For this review, take the finished solid that the model builds, in its own axes (mm). Face numbers are marked on the shaded views. Round coordinates to 2 decimals unless told otherwise and drop trailing zeros. Order: outer loops, then holes, each group sorted by start corner. A loop starts at its lowest first (then second) coordinate and runs counter-clockwise, first axis right, second up. Notation, with made-up numbers: (18, -9) -> (43, -9) arc R16 cw to (43, 14) -> close; hole circle Ø5 at (50, 34.5). An arc over 180 degrees is marked (long way). Use a Markdown table: item, result. Add a question column.
1) Consider section C-C (x = 6.8). State the section outline as (y, z) points, plus the area to 3 significant figures.
2) Consider section D-D (z = 13). State the section outline as (x, y) points.
3) Draft analysis for pull direction X (two halves, no side actions). For the marked faces 1, 2 and 3, state which applies: pulls with the +X half, pulls with the -X half, needs draft (parallel to the pull), parting line crosses it, or undercut.
4) Consider section B-B (y = 1.35). State the section outline as (x, z) points.
5) Wall thickness on line 1 along Z through (x, y) = (8, 1.65); line 2 along Z through (x, y) = (5, 2.5); line 3 along Z through (x, y) = (5.5, 0.5): over which ranges is each line inside the solid? List them lowest first. Write a range as [from, to].
6) Clearance check with a flat-ended pin moving along its axis: P1, Ø1.8, axis at x = 7.3, z = 7.68, coming from the +Y side. State where the tip first meets the part, or that it passes through.
7) Consider section A-A (z = 18.32). State the section outline as (x, y) points.
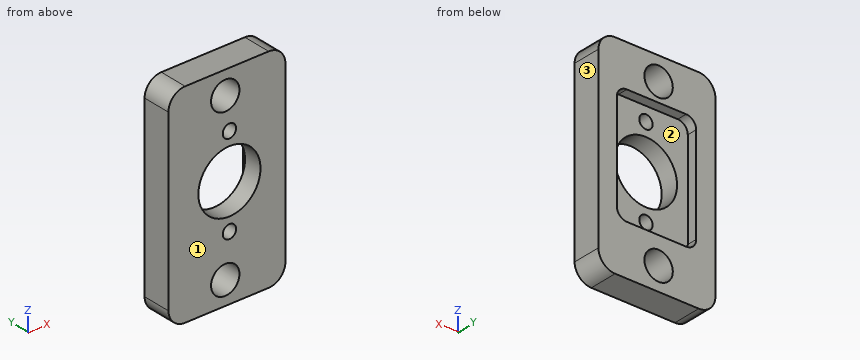
```python
from build123d import *

# Parameters (mm, degrees)
BOSS_EXTRUDE1_DEPTH = 3.4
CUT_EXTRUDE1_DEPTH  = 1.2
SKETCH3_R           = 3.72
SKETCH3_R_2         = 0.8
CUT_EXTRUDE2_DEPTH  = 29.737432036
SKETCH4_R           = 1.7
CUT_EXTRUDE3_DEPTH  = 29.854115824


with BuildPart() as part:
    # Sketch1 → Boss-Extrude1 (new body)
    with BuildSketch(Plane(origin=(0, 0, 0), x_dir=(1, 0, 0), z_dir=(0, 1, 0))):
        with BuildLine():
            Line((2, 0), (12, 0))
            ThreePointArc((12, 0), (13.414213562, -0.585786438), (14, -2))
            Line((14, -2), (14, -23))
            ThreePointArc((14, -23), (13.414213562, -24.414213562), (12, -25))
            Line((12, -25), (2, -25))
            ThreePointArc((2, -25), (0.585786438, -24.414213562), (0, -23))
            Line((0, -23), (0, -2))
            ThreePointArc((0, -2), (0.585786438, -0.585786438), (2, 0))
        make_face()
    extrude(amount=BOSS_EXTRUDE1_DEPTH)

    # Sketch2 → Cut-Extrude1 (cut)
    with BuildSketch(Plane(origin=(0, 3.4, 0), x_dir=(1, 0, 0), z_dir=(0, 1, 0))):
        with BuildLine():
            Line((3.5, -6), (10.6, -6))
            ThreePointArc((10.6, -6), (11.448528137, -6.351471863), (11.8, -7.2))
            Line((11.8, -7.2), (11.8, -18.8))
            ThreePointArc((11.8, -18.8), (11.448528137, -19.648528137), (10.6, -20))
            Line((10.6, -20), (3.5, -20))
            ThreePointArc((3.5, -20), (2.651471863, -19.648528137), (2.3, -18.8))
            Line((2.3, -18.8), (2.3, -7.2))
            ThreePointArc((2.3, -7.2), (2.651471863, -6.351471863), (3.5, -6))
        make_face()
    extrude(amount=-CUT_EXTRUDE1_DEPTH, mode=Mode.SUBTRACT)

    # Sketch3 → Cut-Extrude2 (cut, through all)
    with BuildSketch(Plane(origin=(0, 2.2, 0), x_dir=(1, 0, 0), z_dir=(0, 1, 0))):
        with Locations(Location((7.3, -13, 0), (0, 0, 270))):
            Circle(SKETCH3_R)
        with Locations(Location((7.3, -7.68, 0), (0, 0, 270))):
            Circle(SKETCH3_R_2)
        with Locations(Location((7.3, -18.32, 0), (0, 0, 270))):
            Circle(SKETCH3_R_2)
    extrude(amount=-CUT_EXTRUDE2_DEPTH, mode=Mode.SUBTRACT)

    # Sketch4 → Cut-Extrude3 (cut, through all)
    with BuildSketch(Plane(origin=(0, 3.4, 0), x_dir=(1, 0, 0), z_dir=(0, 1, 0))):
        with Locations(Location((6.8, -2.76, 0), (0, 0, 270))):
            Circle(SKETCH4_R)
        with Locations(Location((6.8, -22.24, 0), (0, 0, 90))):
            Circle(SKETCH4_R)
    extrude(amount=-CUT_EXTRUDE3_DEPTH, mode=Mode.SUBTRACT)


solid = part.part
```
Results list:
| question | item | result |
|---|---|---|
| 1 | outline | (0, 0) -> (3.4, 0) -> (3.4, 1.06) -> (0, 1.06) -> close; (0, 4.46) -> (3.4, 4.46) -> (3.4, 6) -> (2.2, 6) -> (2.2, 7.06) -> (0, 7.06) -> close; (0, 8.3) -> (2.2, 8.3) -> (2.2, 9.31) -> (0, 9.31) -> close; (0, 16.69) -> (2.2, 16.69) -> (2.2, 17.7) -> (0, 17.7) -> close; (0, 18.94) -> (2.2, 18.94) -> (2.2, 20) -> (3.4, 20) -> (3.4, 20.54) -> (0, 20.54) -> close; (0, 23.94) -> (3.4, 23.94) -> (3.4, 25) -> (0, 25) -> close |
| 1 | area | 23.4 mm2 |
| 2 | outline | (0, 0) -> (3.58, 0) -> (3.58, 2.2) -> (2.3, 2.2) -> (2.3, 3.4) -> (0, 3.4) -> close; (11.02, 0) -> (14, 0) -> (14, 3.4) -> (11.8, 3.4) -> (11.8, 2.2) -> (11.02, 2.2) -> close |
| 3 | face 1 | needs draft |
| 3 | face 2 | undercut |
| 3 | face 3 | pulls with the +X half |
| 4 | outline | (0, 2) arc R2 ccw to (2, 0) -> (12, 0) arc R2 ccw to (14, 2) -> (14, 23) arc R2 ccw to (12, 25) -> (2, 25) arc R2 ccw to (0, 23) -> close; hole circle Ø7.44 at (7.3, 13); hole circle Ø3.4 at (6.8, 2.76); hole circle Ø3.4 at (6.8, 22.24); hole circle Ø1.6 at (7.3, 7.68); hole circle Ø1.6 at (7.3, 18.32) |
| 5 | line 1 | [0, 1.56], [3.96, 7.29], [8.07, 9.35], [16.65, 17.93], [18.71, 21.04], [23.44, 25] |
| 5 | line 2 | [0, 6], [20, 25] |
| 5 | line 3 | [0, 1.66], [3.86, 9.74], [16.26, 21.14], [23.34, 25] |
| 6 | P1 | y = 2.2 |
| 7 | outline | (0, 0) -> (6.5, 0) -> (6.5, 2.2) -> (2.3, 2.2) -> (2.3, 3.4) -> (0, 3.4) -> close; (8.1, 0) -> (14, 0) -> (14, 3.4) -> (11.8, 3.4) -> (11.8, 2.2) -> (8.1, 2.2) -> close |
